from build123d import *

# Parameters (mm, degrees)
F3_DEPTH = 12.7
F5_DEPTH = 6.35
F7_D     = 19.05
F8_R     = 1.5875
F9_DEPTH = 3.175


with BuildPart() as f1:
    # F0 (on Front) → F1 (revolve)
    with BuildSketch(Plane.XZ):
        Polygon((0, 0), (31.75, 0), (31.75, 12.7), (38.1, 12.7), (38.1, 38.1), (0, 38.1), align=None)
    revolve(axis=Axis((0, 0, 19.05), (0, 0, -1)))

    # F2 (on face) → F3 (cut)
    with BuildSketch(Plane(origin=(0, 0, 0), x_dir=(1, 0, 0), z_dir=(0, 0, -1))):
        with BuildLine():
            Line((11.4793549074, 25.4), (12.7619952542, 29.0722200241))
            Line((12.7619952542, 29.0722200241), (20.2202573419, 33.7093167499))
            Line((20.2202573419, 33.7093167499), (-32.5390584767, 29.2297520235))
            Line((-32.5390584767, 29.2297520235), (-48.7152673304, -19.05))
            Line((-48.7152673304, -19.05), (-26.924, -19.05))
            Line((-26.924, -19.05), (-26.924, -5.08))
            ThreePointArc((-26.924, -5.08), (-21.844, 0), (-26.924, 5.08))
            Line((-26.924, 5.08), (-26.924, 6.35))
            ThreePointArc((-26.924, 6.35), (-21.3443841816, 19.8203841816), (-7.874, 25.4))
            Line((-7.874, 25.4), (11.4793549074, 25.4))
        make_face()
    extrude(amount=-F3_DEPTH, mode=Mode.SUBTRACT)

    # F4 (on face) → F5 (cut)
    with BuildSketch(Plane(origin=(0, 0, 0), x_dir=(1, 0, 0), z_dir=(0, 0, -1))):
        with BuildLine():
            ThreePointArc((23.868192568, -8.6873116405), (10.7345038482, -23.0202177907), (-8.6873116405, -23.868192568))
            ThreePointArc((-8.6873116405, -23.868192568), (-11.1150385766, -23.9741894151), (-12.7567496665, -25.7658026839))
            Line((-12.7567496665, -25.7658026839), (-28.8802481167, -70.0647505985))
            Line((-28.8802481167, -70.0647505985), (61.9316732098, -19.1625211791))
            Line((61.9316732098, -19.1625211791), (27.937630594, -6.7897015245))
            ThreePointArc((27.937630594, -6.7897015245), (25.5099036579, -6.8956983717), (23.868192568, -8.6873116405))
        make_face()
    extrude(amount=-F5_DEPTH, mode=Mode.SUBTRACT)

    # F7 (through all)
    with Locations(Plane(origin=(0, 0, 0), x_dir=(1, 0, 0), z_dir=(0, 0, -1))):
        with Locations((0, 0)):
            Hole(F7_D / 2)

    # F8 (on face) → F9 (cut)
    with BuildSketch(Plane(origin=(0, 0, 12.7), x_dir=(1, 0, 0), z_dir=(0, 0, -1))):
        with Locations((-26.924, 0)):
            Circle(F8_R)
    extrude(amount=-F9_DEPTH, mode=Mode.SUBTRACT)


solid = f1.part
Read the model definition and answer for the solid it produces. Units are mm, in the model's axes. A direction names the side the tool comes from. Coordinates: 2 decimals unless noted, no trailing zeros. Loops run counter-clockwise (first coordinate to the right, second up) from the corner with the lowest first, then second, coordinate; pieces in that order, holes last.
Q1. Each of these flat-tipped pins is pushed along its axis until it touches: pin 1 Ø3.5 at (y, z) = (8.5, 8) entering from -X; pin 2 Ø4 at (y, z) = (-13.5, 23) entering from -X; pin 3 Ø6.5 at (x, z) = (4.5, 4) entering from -Y. Where does it stop, or does it pass through?
Q2. The part is cut by section D-D on x = 25.5. Write down the section's boundary in (y, z).
Q3. Consider probe 1 along Y at (x, z) = (0, 25) (3 decimals); probe 2 along Y at (x, z) = (-7, 33.5); probe 3 along Y at (x, z) = (-18, 13). Determine where each line is inside the solid, lowest interval first.
Q4. The part is cut by section C-C on z = 10.5. Write down the section's boundary in (x, y) (3 decimals), and give its area (3 significant figures).
Q5. The part is cut by section A-A on x = 0. Write down the section's boundary in (y, z) (3 decimals), and give its area (3 significant figures).
Q6. The mould has two halves that part along X. Classify faces 1 (the face through (-13.265, 27.163, 3.131)), 2 (the face through (2, -25.4, 6)), 3 (the face through (25.5, 6.9, 3.1)): +X half, -X half, draft (parallel to the pull), parting line (faces both ways), or undercut.
Q7. Which of the six approach directions +Z, -Z, +X, -X, +Y, -Y give full straight-line access (tool end or side, diameter ignored) to faces 4 (the face through (-11.08, 23.96, 3.13)), 5 (the face through (-27, 0, 15.875)), 6 (the face through (-21.845, 0.112, 6.261)), 7 (the face through (8, 8, 38.1)), 8 (the face through (-21.492, -19.671, 6.261))?
Results below:
1. pin 1: stops at x = -26.92
1. pin 2: stops at x = -36.32
1. pin 3: stops at y = -25.4
2. outline: (-28.31, 12.7) - (-18.92, 12.7) - (-18.92, 0) - (6.9, 0) - (6.9, 6.35) - (18.92, 6.35) - (18.92, 12.7) - (28.31, 12.7) - (28.31, 38.1) - (-28.31, 38.1) - close
3. probe 1: y = -38.1 to -9.525, 9.525 to 38.1
3. probe 2: y = -37.45 to -6.46, 6.46 to 37.45
3. probe 3: y = -33.58 to 33.58
4. outline: (-26.924, -6.35) arc R19.05 ccw to (-7.874, -25.4) - (11.479, -25.4) - (12.762, -29.072) arc R31.75 ccw (long way) to (-26.924, 16.827) - (-26.924, 5.08) arc R5.08 cw to (-26.924, -5.08) - close; hole circle Ø19.05 at (0, 0)
4. area: 2,530 mm2
5. outline: (-38.1, 12.7) - (-25.4, 12.7) - (-25.4, 0) - (-9.525, 0) - (-9.525, 38.1) - (-38.1, 38.1) - close; (9.525, 0) - (25.4, 0) - (25.4, 6.35) - (31.75, 6.35) - (31.75, 12.7) - (38.1, 12.7) - (38.1, 38.1) - (9.525, 38.1) - close
5. area: 1,900 mm2
6. face 1: +X half
6. face 2: draft
6. face 3: undercut
7. face 4: -Z, +Y
7. face 5: -Z
7. face 6: -Z, -X
7. face 7: +Z, +X, -X, +Y, -Y
7. face 8: -Z, -X, -Y
